Input: dimensioned drawing with shaded views. Units: mm. Origin: part minimum x, y, z. A direction names the side the tool comes from. Give positions to 0.01 mm unless a question says otherwise; leave off trailing zeros. Loops run counter-clockwise (first coordinate to the right, second up) from the corner with the lowest first, then second, coordinate; pieces in that order, holes last.
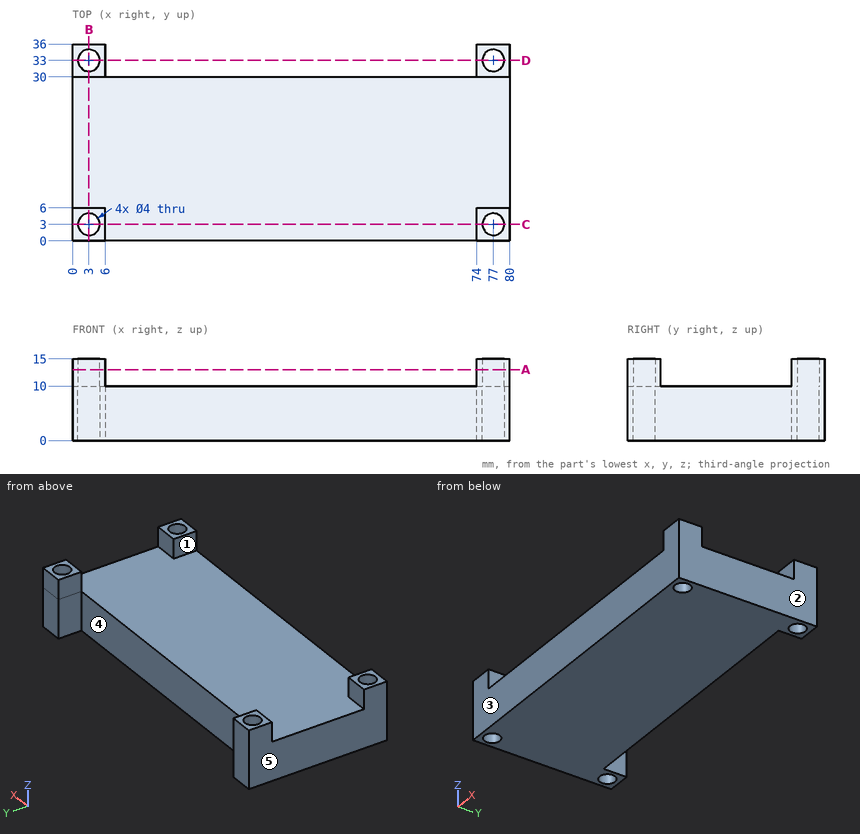
(1) Section D-D, the plane y = 33. Return the cut outline in (x, z), then the cut area to 3 significant figures.
A:
outline: (0, 0) - (1, 0) - (1, 15) - (0, 15) - close; (5, 0) - (6, 0) - (6, 15) - (5, 15) - close; (74, 0) - (75, 0) - (75, 15) - (74, 15) - close; (79, 0) - (80, 0) - (80, 15) - (79, 15) - close
area: 60.0 mm2
(2) Section C-C, the plane y = 3. Return the cut outline in (x, z), then the cut area to 3 significant figures.
A:
outline: (0, 0) - (1, 0) - (1, 15) - (0, 15) - close; (5, 0) - (75, 0) - (75, 15) - (74, 15) - (74, 10) - (6, 10) - (6, 15) - (5, 15) - close; (79, 0) - (80, 0) - (80, 15) - (79, 15) - close
area: 740 mm2
(3) Ray query, line 1 along Y through (x, z) = (3, 13.9); line 2 along Y through (x, z) = (77, 4.25); line 3 along X through (y, z) = (34, 9.5). Return the intervals inside material, ascending.
A:
line 1: y = 0 to 1, 5 to 6, 30 to 31, 35 to 36
line 2: y = 0 to 1, 5 to 31, 35 to 36
line 3: x = 0 to 1.27, 4.73 to 6, 74 to 75.27, 78.73 to 80
(4) Mould query, pull axis X, two halves, no side actions, for the marked faces 3, 4 and 5. Classes: pulls with the +X half, pulls with the -X half, needs draft (parallel to the pull), parting line crosses it, or undercut.
A:
face 3: needs draft
face 4: undercut
face 5: pulls with the -X half
(5) Section A-A, the plane z = 13. Return the cut outline in (x, y), then the cut area to 3 significant figures.
A:
outline: (0, 0) - (6, 0) - (6, 6) - (0, 6) - close; (0, 30) - (6, 30) - (6, 36) - (0, 36) - close; (74, 0) - (80, 0) - (80, 6) - (74, 6) - close; (74, 30) - (80, 30) - (80, 36) - (74, 36) - close; hole circle Ø4 at (3, 3); hole circle Ø4 at (3, 33); hole circle Ø4 at (77, 3); hole circle Ø4 at (77, 33)
area: 93.7 mm2
(6) Reachability of the marked faces 1 and 2 from +Z, -Z, +X, -X, +Y, -Y: full face, straight path, thin tool, end or side. Return the list, or none.
A:
face 1: +Z, +Y, -Y
face 2: +Z, -Z, +X, +Y, -Y
(7) First-contact query: pin 1 (3.5 mm diameter, centred on x = 77, y = 33, fed in from +Z); pin 2 (8 mm diameter, centred on x = 58.5, z = 7, fed in from +Y). Flat tips, straight axial feed; report the tip coordinate or a pass-through.
A:
pin 1: passes through
pin 2: stops at y = 30
(8) Section B-B, the plane x = 3. Return the cut outline in (y, z), then the cut area to 3 significant figures.
A:
outline: (0, 0) - (1, 0) - (1, 15) - (0, 15) - close; (5, 0) - (31, 0) - (31, 15) - (30, 15) - (30, 10) - (6, 10) - (6, 15) - (5, 15) - close; (35, 0) - (36, 0) - (36, 15) - (35, 15) - close
area: 300 mm2
